Verification items for this drawing (mm, ordinates from the low corner). A direction names the side the tool comes from. Coordinates: 2 decimals unless noted, no trailing zeros. Write each loop counter-clockwise with the first axis right and the second up, starting at its lowest first coordinate (ties: lowest second). Pieces come first, ordered by that corner, then holes. Notation, with made-up numbers: (35, 21.25) -> (47, 21.25) arc R7 ccw to (47, 32.25) -> close; hole circle Ø5 at (30, 4.5). An arc over 180 degrees is marked (long way). One line per question, with ' | ' between items.
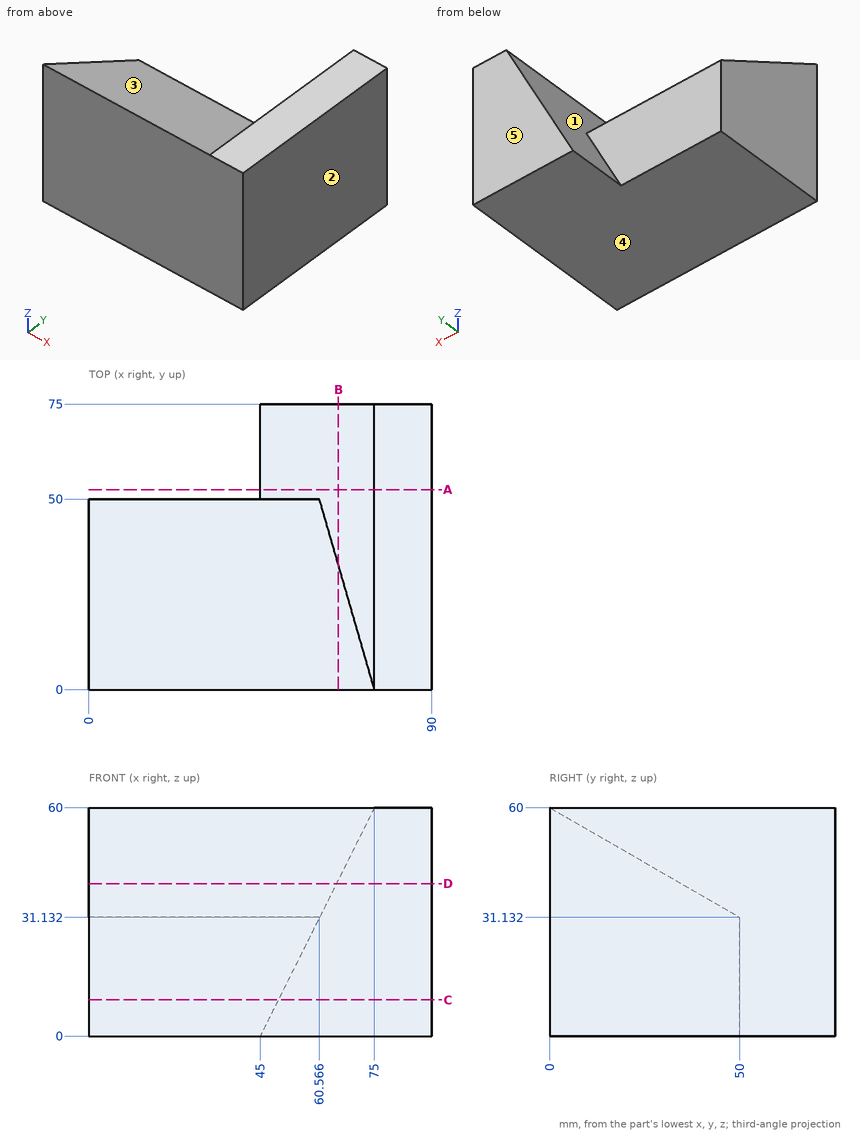
(1) Depth check by flat-ended pin: P1, Ø2, axis at x = 41.5, z = 8, coming from the +Y side. Enter the tip coordinate at first touch or a pass-through.
Answers below:
P1: stops at y = 50
(2) Material ranges on line 1 (Y direction, x = 41, z = 16); line 2 (Y direction, x = 32.5, z = 44) (1 decimal); line 3 (Z direction, x = 7, y = 17) (1 decimal), recorded low to high.
Answers below:
line 1: y = 0 to 50 | line 2: y = 0 to 27.7 | line 3: z = 0 to 50.2
(3) Cross-section at D-D (z = 40). Record the cut outline in (x, y), plus the area to 3 significant figures.
Answers below:
outline: (0, 0) -> (90, 0) -> (90, 75) -> (65, 75) -> (65, 34.64) -> (0, 34.64) -> close | area: 4,130 mm²
(4) Cross-section at B-B (x = 65.5). Record the cut outline in (y, z), plus the area to 3 significant figures.
Answers below:
outline: (0, 0) -> (75, 0) -> (75, 41) -> (32.91, 41) -> (0, 60) -> close | area: 3,390 mm²
(5) Tool access check on the marked faces 1 and 2. Record the directions out of +Z, -Z, +X, -X, +Y, -Y that give a thin tool (end or side, any length) a straight path to the whole face; none if there is none.
Answers below:
face 1: +Z, -X, +Y | face 2: +Z, -Z, +X, +Y, -Y
(6) Draft check along Z on the marked faces 3, 4 and 5. Enter one of: pulls with the +Z half, pulls with the -Z half, needs draft (parallel to the pull), parting line crosses it, or undercut.
Answers below:
face 3: pulls with the +Z half | face 4: pulls with the -Z half | face 5: needs draft
(7) Cross-section at A-A (y = 52.5). Record the cut outline in (x, z), plus the area to 3 significant figures.
Answers below:
outline: (45, 0) -> (90, 0) -> (90, 60) -> (75, 60) -> close | area: 1,800 mm²
(8) Cross-section at C-C (z = 9.5). Record the cut outline in (x, y).
Answers below:
outline: (0, 0) -> (90, 0) -> (90, 75) -> (49.75, 75) -> (49.75, 50) -> (0, 50) -> close
